The model under review builds one solid part; all positions refer to its coordinate system, in mm. A direction names the side the tool comes from. Coordinates: 2 decimals unless noted, no trailing zeros. Order: outer loops, then holes, each group sorted by start corner. A loop starts at its lowest first (then second) coordinate and runs counter-clockwise, first axis right, second up. Notation, with made-up numbers: (76.25, 70.25) -> (102.25, 70.25) arc R10 cw to (102.25, 85.25) -> close; hole circle Ø1 at (17.25, -15.75). An arc over 180 degrees is marked (long way). Put each result on its own line as item: value.
from build123d import *

# Parameters (mm, degrees)
SKETCH1_R           = 6.35
BOSS_EXTRUDE1_DEPTH = 577.85
BOSS_EXTRUDE2_START = 25.4
BOSS_EXTRUDE2_DEPTH = 11.049


with BuildPart() as part:
    # Sketch1 → Boss-Extrude1 (new body)
    with BuildSketch(Plane(origin=(0, 0, 0), x_dir=(1, 0, 0), z_dir=(0, 1, 0))):
        Circle(SKETCH1_R)
    extrude(amount=BOSS_EXTRUDE1_DEPTH)

    # Sketch3 → Boss-Extrude2 (add)
    with BuildSketch(Plane(origin=(0, 0, 0), x_dir=(1, 0, 0), z_dir=(0, 1, 0)).offset(BOSS_EXTRUDE2_START)):
        Polygon((9.876865428, 4.838907863), (0.747815578, 10.973070302), (-9.129049851, 6.134162439), (-9.876865428, -4.838907863), (-0.747815578, -10.973070302), (9.129049851, -6.134162439), align=None)
    extrude(amount=BOSS_EXTRUDE2_DEPTH)


solid = part.part
Item 1: For line 1 (Y direction, x = 8, z = 5.5); line 2 (Z direction, x = -2, y = 417.5); line 3 (Z direction, x = 0, y = 95), list the stretches that pass through material, from the lowest coordinate up. Write a range as from..to.
Answers below:
line 1: 25.4..36.45
line 2: -6.03..6.03
line 3: -6.35..6.35
Item 2: For faces 1 (the flat face through (-5, 36.449, 5)), 2 (the flat face through (5.38, 30.85, -7.86)), 3 (the cylindrical face through (-1.38, 12.52, 6.2)), list the 3-axis set-ups (+Z, -Z, +X, -X, +Y, -Y) from which the entire face can be reached by the end or side of a thin tool; tool diameter is ignored.
Answers below:
face 1: +Y
face 2: -Z, +X, +Y, -Y
face 3: -Y
Item 3: Consider section B-B on z = 0. Write out the cut boundary in (x, y).
Answers below:
outline: (-9.55, 25.4) -> (-6.35, 25.4) -> (-6.35, 0) -> (6.35, 0) -> (6.35, 25.4) -> (9.55, 25.4) -> (9.55, 36.45) -> (6.35, 36.45) -> (6.35, 577.85) -> (-6.35, 577.85) -> (-6.35, 36.45) -> (-9.55, 36.45) -> close
Item 4: Consider section A-A on y = 352. Write out the cut boundary in (x, z).
Answers below:
outline: circle Ø12.7 at (0, 0)
Item 5: For pin 1 Ø4 at (x, z) = (5, -7.5) entering from +Y; pin 2 Ø3 at (y, z) = (236.5, 1) entering from +X; pin 3 Ø1 at (x, y) = (3, 446) entering from -Z, all flat-tipped, find the tip position at first contact; note any pin that passes through.
Answers below:
pin 1: y = 36.45
pin 2: x = 6.35
pin 3: z = -5.84
